```python
from build123d import *

# Parameters (mm, degrees)
IZIM1_R                     = 7.5
IZIM1_R_2                   = 2.75
Y_KSEKLIK_EKSTR_ZYON1_DEPTH = 15
IZIM2_R                     = 7.5
IZIM2_R_2                   = 4.25
Y_KSEKLIK_EKSTR_ZYON2_DEPTH = 30
IZIM3_R                     = 1.5
KES_EKSTR_ZYON1_DEPTH       = 30


with BuildPart() as part:
    # Çizim1 → Yükseklik-Ekstrüzyon1 (new body)
    with BuildSketch(Plane(origin=(0, 0, 0), x_dir=(1, 0, 0), z_dir=(0, 1, 0))):
        with Locations(Location((0, 0, 0), (0, 0, 270))):
            Circle(IZIM1_R)
        with Locations(Location((0, 0, 0), (0, 0, 270))):
            Circle(IZIM1_R_2, mode=Mode.SUBTRACT)
    extrude(amount=Y_KSEKLIK_EKSTR_ZYON1_DEPTH)

    # Çizim2 → Yükseklik-Ekstrüzyon2 (add)
    with BuildSketch(Plane(origin=(0, 15, 0), x_dir=(1, 0, 0), z_dir=(0, 1, 0))):
        with Locations(Location((0, 0, 0), (0, 0, 270))):
            Circle(IZIM2_R)
        with Locations(Location((0, 0, 0), (0, 0, 270))):
            Circle(IZIM2_R_2, mode=Mode.SUBTRACT)
    extrude(amount=Y_KSEKLIK_EKSTR_ZYON2_DEPTH)

    # Çizim3 → Kes-Ekstrüzyon1 (cut)
    with BuildSketch(Plane.XY):
        with Locations(Location((0, 40, 0), (0, 0, 90))):
            Circle(IZIM3_R)
        with Locations(Location((0, 35, 0), (0, 0, 90))):
            Circle(IZIM3_R)
        with Locations(Location((0, 30, 0), (0, 0, 90))):
            Circle(IZIM3_R)
        with Locations(Location((0, 9, 0), (0, 0, 90))):
            Circle(IZIM3_R)
        with Locations(Location((0, 4, 0), (0, 0, 90))):
            Circle(IZIM3_R)
    extrude(amount=-KES_EKSTR_ZYON1_DEPTH, mode=Mode.SUBTRACT)


solid = part.part
```
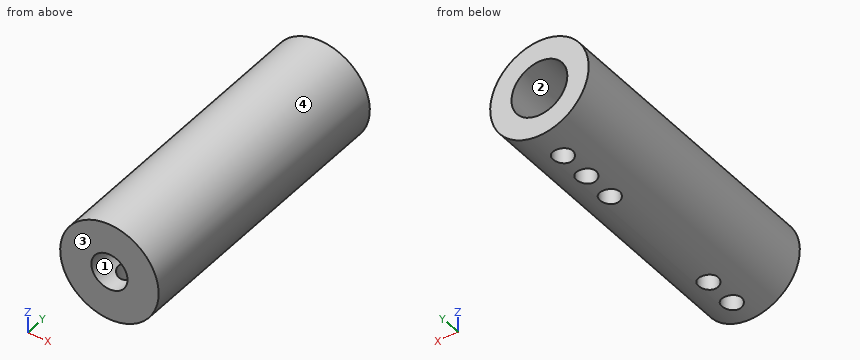
Source: CAD feature listing. Evaluate the final solid. Frame: model axes, mm. Face numbers are marked on the shaded views. Give positions to 0.01 mm unless a question says otherwise; leave off trailing zeros. Order: outer loops, then holes, each group sorted by start corner. A loop starts at its lowest first (then second) coordinate and runs counter-clockwise, first axis right, second up.
(1) Contact query for flat-ended pins moving along their axis: P1, Ø5, axis at x = 0, y = 35, coming from the -Z side; P2, Ø2, axis at y = 8.5, z = -3.5, coming from the +X side; P3, Ø1.8, axis at x = 0, y = 40, coming from the -Z side; P4, Ø5, axis at x = 0, z = 0, coming from the +Y side. Output: stop coordinate, or through.
(2) Material intervals for line 1 along Z through (x, y) = (0, 32.5); line 2 along Y through (x, z) = (3.75, 1.75), sorted ascending.
(3) Section query A-A (z = 0). Return the cut outline in (x, y), plus the area to 4 significant figures.
(4) Pull-direction query (X, two-part tool) for the marked faces 1, 2, 3 and 4; classes: +X half, -X half, draft (parallel to the pull), parting line (faces both ways), or undercut.
(5) Section query D-D (x = 2). Return the cut outline in (y, z), plus the area to 3 significant figures.
(6) Section query C-C (y = 11). Return the cut outline in (x, z), plus the area to 3 significant figures.
(7) Section query B-B (x = 0). State how many separate pieces and enclosed holes the cut face has, plus the area to 3 significant figures.
Outcome:
1. P1: stops at z = -7.5
1. P2: stops at x = 7.07
1. P3: stops at z = 4.15
1. P4: passes through
2. line 1: z = -7.5 to -4.25, 4.25 to 7.5
2. line 2: y = 0 to 15
3. outline: (-7.5, 0) - (-2.75, 0) - (-2.75, 15) - (-4.25, 15) - (-4.25, 45) - (-7.5, 45) - close; (2.75, 0) - (7.5, 0) - (7.5, 45) - (4.25, 45) - (4.25, 15) - (2.75, 15) - close
3. area: 337.5 mm2
4. face 1: undercut
4. face 2: undercut
4. face 3: draft
4. face 4: parting line
5. outline: (0, -7.23) - (45, -7.23) - (45, -3.75) - (15, -3.75) - (15, -1.89) - (0, -1.89) - close; (0, 1.89) - (15, 1.89) - (15, 3.75) - (45, 3.75) - (45, 7.23) - (0, 7.23) - close
5. area: 369 mm2
6. outline: circle Ø15 at (0, 0); hole circle Ø5.5 at (0, 0)
6. area: 153 mm2
7. separate pieces: 7
7. enclosed holes: 0
7. area: 280 mm2
